```python
from build123d import *

# Parameters (mm, degrees)
F0_R     = 2.25
F1_DEPTH = 25
F3_DEPTH = 40.001
F4_R     = 2.25
F5_DEPTH = 20.001
F6_R     = 5
F7_R     = 1
F8_R     = 1


with BuildPart() as f1:
    # F0 (on Top) → F1 (new body)
    with BuildSketch(Plane.XY):
        Polygon((-113.1, -20), (113.1, -20), (113.1, 0), (60.5, 0), (60.5, 20), (-113.1, 20), align=None)
        with Locations((-99.6, 0)):
            Circle(F0_R, mode=Mode.SUBTRACT)
    extrude(amount=F1_DEPTH)

    # F2 (on face) → F3 (cut, through all)
    with BuildSketch(Plane.XZ.offset(20)):
        with BuildLine():
            Line((-45.1, 30), (-95.5, 30))
            ThreePointArc((-95.5, 30), (-70.3, 4.8), (-45.1, 30))
        make_face()
        with BuildLine():
            Line((7.3, 30), (-43.1, 30))
            ThreePointArc((-43.1, 30), (-17.9, 4.8), (7.3, 30))
        make_face()
        with BuildLine():
            Line((59.7, 30), (9.3, 30))
            ThreePointArc((9.3, 30), (34.5, 4.8), (59.7, 30))
        make_face()
        with BuildLine():
            Line((112.1, 30), (61.7, 30))
            ThreePointArc((61.7, 30), (86.9, 4.8), (112.1, 30))
        make_face()
    extrude(amount=-F3_DEPTH, mode=Mode.SUBTRACT)

    # F4 (on face) → F5 (cut, through all)
    with BuildSketch(Plane(origin=(0, 0, 0), x_dir=(-1, 0, 0), z_dir=(0, 1, 0))):
        with Locations((-66.9, 5)):
            Circle(F4_R)
        with Locations((-106.9, 5)):
            Circle(F4_R)
    extrude(amount=-F5_DEPTH, mode=Mode.SUBTRACT)

    # F6
    f6_edges = [f1.edges().sort_by_distance(p)[0] for p in [
        (-113.1, 0, 25),
    ]]
    fillet(f6_edges, radius=F6_R)

    # F7
    f7_edges = [f1.edges().sort_by_distance(p)[0] for p in [
        (113.1, 0, 12.5),
    ]]
    fillet(f7_edges, radius=F7_R)

    # F8
    f8_edges = [f1.edges().sort_by_distance(p)[0] for p in [
        (-113.1, 20, 10),
        (-111.635534, 20, 23.535534),
        (-101.549494, 20, 25),
        (-113.1, -20, 10),
        (-111.635534, -20, 23.535534),
        (-101.549494, -20, 25),
    ]]
    fillet(f8_edges, radius=F8_R)


solid = f1.part
```
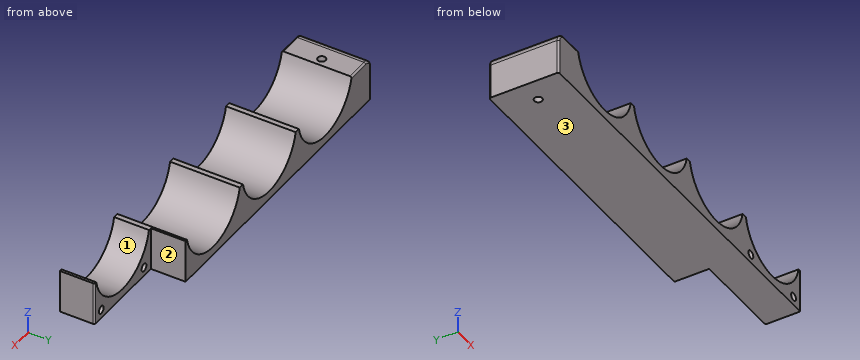
Input: part model. Units: mm. Frame: model coordinates. Face numbers are marked on the shaded views. Round coordinates to 2 decimals unless told otherwise and drop trailing zeros. Loops run counter-clockwise (first coordinate to the right, second up) from the corner with the lowest first, then second, coordinate; pieces in that order, holes last. Notation, with made-up numbers: (-4, 44.25) - (19, 44.25) arc R18 cw to (19, 63.25) - close; hole circle Ø2 at (-20, 52). An arc over 180 degrees is marked (long way). One line per item, written item: value. Start each with the question number.
(1) Section C-C, the plane x = -99.6. Return loops of the section in (y, z).
(2) Section D-D, the plane y = 16. Return loops of the section in (x, z), plus the area to 3 significant figures.
(3) Section A-A, the plane z = 15.5. Return loops of the section in (x, y), plus the area to 3 significant figures.
(4) Draft query along X for the marked faces 1, 2 and 3. Return one class per face: +X half, -X half, draft (parallel to the pull), parting line (faces both ways), or undercut.
(5) Section B-B, the plane y = -11. Return loops of the section in (x, z), plus the area to 3 significant figures.
(6) Ray query, line 1 (X direction, y = -4.5, z = 4.75); line 2 (X direction, y = 5, z = 21.25); line 3 (X direction, y = -13, z = 9.25). Return the intervals inside material, ascending. Write a range as [from, to].
(7) Contact query for flat-ended pins moving along their axis: P1, Ø6, axis at y = 15, z = 8, coming from the +X side; P2, Ø12.5, axis at x = 99, z = 14, coming from the +Y side; P3, Ø1, axis at x = -40.5, y = 0.5, coming from the +Z side. Output: stop coordinate, or through.
Results below:
1. outline: (-20, 0) - (-2.25, 0) - (-2.25, 25) - (-19, 25) arc R1 ccw to (-20, 24) - close; (2.25, 0) - (20, 0) - (20, 24) arc R1 ccw to (19, 25) - (2.25, 25) - close
2. outline: (-113.1, 0) - (60.5, 0) - (60.5, 25) - (59.2, 25) arc R25.2 cw to (9.8, 25) - (6.8, 25) arc R25.2 cw to (-42.6, 25) - (-45.6, 25) arc R25.2 cw to (-95, 25) - (-108.1, 25) arc R5 ccw to (-113.1, 20) - close
2. area: 2,090 mm^2
3. outline: (-113.1, -19) arc R1 ccw to (-112.1, -20) - (-90.91, -20) - (-90.91, 20) - (-112.1, 20) arc R1 ccw to (-113.1, 19) - close; (-49.69, -20) - (-38.51, -20) - (-38.51, 20) - (-49.69, 20) - close; (2.71, -20) - (13.89, -20) - (13.89, 20) - (2.71, 20) - close; (55.11, -20) - (66.29, -20) - (66.29, 0) - (60.5, 0) - (60.5, 20) - (55.11, 20) - close; (107.51, -20) - (113.1, -20) - (113.1, -1) arc R1 ccw to (112.1, 0) - (107.51, 0) - close; hole circle Ø4.5 at (-99.6, 0)
3. area: 2,210 mm^2
4. face 1: undercut
4. face 2: +X half
4. face 3: draft
5. outline: (-113.1, 0) - (113.1, 0) - (113.1, 25) - (111.6, 25) arc R25.2 cw to (62.2, 25) - (59.2, 25) arc R25.2 cw to (9.8, 25) - (6.8, 25) arc R25.2 cw to (-42.6, 25) - (-45.6, 25) arc R25.2 cw to (-95, 25) - (-108.1, 25) arc R5 ccw to (-113.1, 20) - close; hole circle Ø4.5 at (66.9, 5); hole circle Ø4.5 at (106.9, 5)
5. area: 2,630 mm^2
6. line 1: [-113.1, 64.66], [69.14, 104.66], [109.14, 113.1]
6. line 2: [-112.94, -93.93], [-46.67, -41.53], [5.73, 10.87], [58.13, 60.5]
6. line 3: [-113.1, -84.6], [-56, -32.2], [-3.6, 20.2], [48.8, 72.6], [101.2, 113.1]
7. P1: x = 60.5
7. P2: y = 0
7. P3: z = 19.93
